Build history of the part. All positions in model axes, mm. Face numbers are marked on the shaded views. A direction names the side the tool comes from. Coordinates: 2 decimals unless noted, no trailing zeros. Order: outer loops, then holes, each group sorted by start corner. A loop starts at its lowest first (then second) coordinate and runs counter-clockwise, first axis right, second up. Notation, with made-up numbers: (-7.75, 63) - (44.25, 63) arc R12 ccw to (44.25, 83) - close; hole circle Ø9 at (38.5, -3). An arc over 180 degrees is marked (long way). Write each question's results on one line, items separated by ' | '. Start each with the question number.
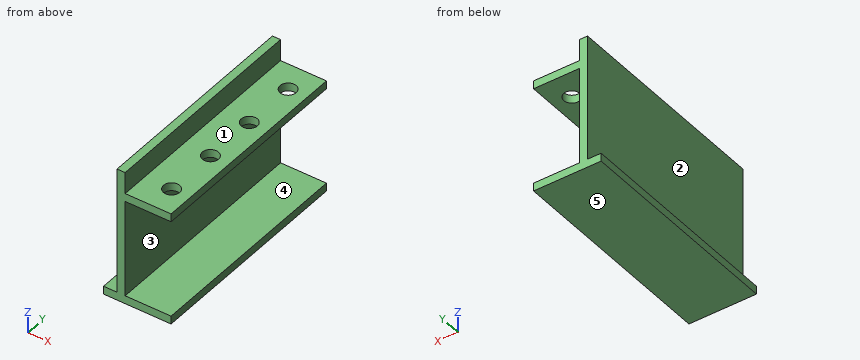
from build123d import *

# Parameters (mm, degrees)
F0_W     = 20
F0_H     = 80
F1_DEPTH = 50
F2_W     = 17
F2_H     = 36
F2_H_2   = 8
F3_DEPTH = 80.001
F4_R     = 3
F5_DEPTH = 3
F6_W     = 5
F6_H     = 3
F7_DEPTH = 80


with BuildPart() as f1:
    # F0 (on Top) → F1 (new body)
    with BuildSketch(Plane.XY):
        Rectangle(F0_W, F0_H)
    extrude(amount=F1_DEPTH)

    # F2 (on face) → F3 (cut, through all)
    with BuildSketch(Plane.XZ.offset(40)):
        with Locations((1.5, 21)):
            Rectangle(F2_W, F2_H)
        with Locations((1.5, 46)):
            Rectangle(F2_W, F2_H_2)
    extrude(amount=-F3_DEPTH, mode=Mode.SUBTRACT)

    # F4 (on face) → F5 (cut, through all)
    with BuildSketch(Plane.XY.offset(42)):
        with Locations((3, -30)):
            Circle(F4_R)
        with Locations((3, -10)):
            Circle(F4_R)
        with Locations((3, 10)):
            Circle(F4_R)
        with Locations((3, 30)):
            Circle(F4_R)
    extrude(amount=-F5_DEPTH, mode=Mode.SUBTRACT)

    # F6 (on face) → F7 (join, through all)
    with BuildSketch(Plane.XZ.offset(40)):
        with Locations((-12.5, 1.5)):
            Rectangle(F6_W, F6_H)
    extrude(amount=-F7_DEPTH)


solid = f1.part
Item 1: Slice it at C-C (z = 17). Write the cut outline in (x, y).
Item 2: Pull direction Z, two halves, no side cores. Call the marked faces 1, 2 and 3: released by +Z, released by -Z, zero draft, split by the parting line, or undercut.
Item 3: Which spindle directions (+Z, -Z, +X, -X, +Y, -Y) get a long thin tool onto all of the face, cutting with end or side? Do the marked faces 4 and 5. Say none if no direction does.
Item 4: Slice it at B-B (y = 20). Write the cut outline in (x, z), then the cut area to 3 significant figures.
Item 5: Flat gauge pins, fed straight in: P1, Ø23.5, axis at y = 12.5, z = 32.5, coming from the -X side; P2, Ø3, axis at x = 2, y = -6, coming from the +Z side; P3, Ø18, axis at y = -15.5, z = 13.5, coming from the +X side. Where does each tip first touch, or does it go through?
Item 6: Probe probe 1 along Y at (x, z) = (3, 39.9); probe 2 along Z at (x, y) = (-5, 31.5); probe 3 along X at (y, z) = (28, 12.5). List the from-to ranges inside material, lowest first.
Item 7: Slice it at A-A (y = 30). Write the cut outline in (x, z).
Item 8: Slice it at D-D (y = 8). Write the cut outline in (x, z).
Resolved:
1) outline: (-10, -40) - (-7, -40) - (-7, 40) - (-10, 40) - close
2) face 1: released by +Z | face 2: zero draft | face 3: undercut
3) face 4: +X, +Y, -Y | face 5: -Z, +X, -X, +Y, -Y
4) outline: (-15, 0) - (10, 0) - (10, 3) - (-7, 3) - (-7, 39) - (10, 39) - (10, 42) - (-7, 42) - (-7, 50) - (-10, 50) - (-10, 3) - (-15, 3) - close | area: 267 mm^2
5) P1: x = -10 | P2: z = 42 | P3: x = -7
6) probe 1: -40 to -33, -27 to -13, -7 to 7, 13 to 27, 33 to 40 | probe 2: 0 to 3, 39 to 42 | probe 3: -10 to -7
7) outline: (-15, 0) - (10, 0) - (10, 3) - (-7, 3) - (-7, 39) - (0, 39) - (0, 42) - (-7, 42) - (-7, 50) - (-10, 50) - (-10, 3) - (-15, 3) - close; (6, 39) - (10, 39) - (10, 42) - (6, 42) - close
8) outline: (-15, 0) - (10, 0) - (10, 3) - (-7, 3) - (-7, 39) - (0.76, 39) - (0.76, 42) - (-7, 42) - (-7, 50) - (-10, 50) - (-10, 3) - (-15, 3) - close; (5.24, 39) - (10, 39) - (10, 42) - (5.24, 42) - close
